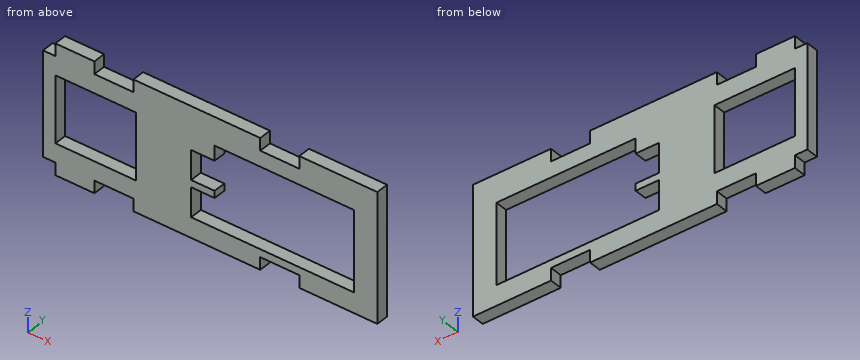
```python
from build123d import *

# Parameters (mm, degrees)
SKETCH1_W           = 20.6
SKETCH1_H           = 17
BOSS_EXTRUDE1_DEPTH = 3.17


with BuildPart() as part:
    # Sketch1 → Boss-Extrude1 (new body)
    with BuildSketch(Plane(origin=(0, 0, 0), x_dir=(1, 0, 0), z_dir=(0, 1, 0))):
        Polygon((55.67, 29.77), (55.67, 32.94), (23.17, 32.94), (23.17, 29.77), (13.17, 29.77), (13.17, 32.94), (3.17, 32.94), (3.17, 29.77), (0, 29.77), (0, 3.17), (3.17, 3.17), (3.17, 0), (13.17, 0), (13.17, 3.17), (23.17, 3.17), (23.17, 0), (55.67, 0), (55.67, 3.17), (65.67, 3.17), (65.67, 0), (85.67, 0), (85.67, 32.94), (65.67, 32.94), (65.67, 29.77), align=None)
        with Locations((13.47, 16.47)):
            Rectangle(SKETCH1_W, SKETCH1_H, mode=Mode.SUBTRACT)
        Polygon((37.97, 27.77), (43.97, 27.77), (79.67, 27.77), (79.67, 7.17), (43.97, 7.17), (43.97, 10.97), (37.97, 10.97), (37.97, 18.47), (43.97, 18.47), (43.97, 20.27), (37.97, 20.27), align=None, mode=Mode.SUBTRACT)
    extrude(amount=-BOSS_EXTRUDE1_DEPTH)


solid = part.part
```
Could you check a few things on this model? Use its own coordinates, in mm. Round coordinates to 2 decimals unless told otherwise and drop trailing zeros. Order: outer loops, then holes, each group sorted by start corner. A loop starts at its lowest first (then second) coordinate and runs counter-clockwise, first axis right, second up. Notation, with made-up numbers: (66, 54.5) -> (94, 54.5) arc R20 ccw to (94, 75.5) -> close; hole circle Ø4 at (-15.5, 48.5). An arc over 180 degrees is marked (long way). One line per question, with ' | ' between items.
Q1. I'm going to push flat-ended pins straight in: pin 1 (1.6 mm diameter, centred on x = 17.5, y = -2.5, fed in from +Z); pin 2 (1 mm diameter, centred on x = 61, y = -1.5, fed in from -Z); pin 3 (1.6 mm diameter, centred on y = -1.5, z = -31, fed in from -X); pin 4 (1.5 mm diameter, centred on y = -2.5, z = -5.5, fed in from -X). Where does each tip first touch, or does it pass through?
Computed values:
pin 1: z = -3.17 | pin 2: z = -29.77 | pin 3: x = 3.17 | pin 4: x = 0
Q2. If we section it at C-C on z = -23.5: Write out the boundary of the cut face in (x, y).
Computed values:
outline: (0, -3.17) -> (3.17, -3.17) -> (3.17, 0) -> (0, 0) -> close; (23.77, -3.17) -> (37.97, -3.17) -> (37.97, 0) -> (23.77, 0) -> close; (79.67, -3.17) -> (85.67, -3.17) -> (85.67, 0) -> (79.67, 0) -> close
Q3. If we section it at D-D on y = -0.9: Give the number of separate pieces and of enclosed holes in the cut face, plus the area to 3 significant figures.
Computed values:
separate pieces: 1 | enclosed holes: 2 | area: 1,500 mm²
Q4. If we section it at B-B on x = 41.5: Write out the boundary of the cut face in (y, z), plus the area to 3 significant figures.
Computed values:
outline: (-3.17, -32.94) -> (0, -32.94) -> (0, -27.77) -> (-3.17, -27.77) -> close; (-3.17, -20.27) -> (0, -20.27) -> (0, -18.47) -> (-3.17, -18.47) -> close; (-3.17, -10.97) -> (0, -10.97) -> (0, 0) -> (-3.17, 0) -> close | area: 56.9 mm²
Q5. If we section it at A-A on x = 18.5: Write out the boundary of the cut face in (y, z).
Computed values:
outline: (-3.17, -29.77) -> (0, -29.77) -> (0, -24.97) -> (-3.17, -24.97) -> close; (-3.17, -7.97) -> (0, -7.97) -> (0, -3.17) -> (-3.17, -3.17) -> close
Q6. If I drill on line 1 (X direction, y = -1.95, z = -24); line 2 (Z direction, x = 41, y = -0.4); line 3 (Z direction, x = 76.5, y = -2.45), over which ranges is the centre line in solid material (lowest first)? Write a range as from..to.
Computed values:
line 1: 0..3.17, 23.77..37.97, 79.67..85.67 | line 2: -32.94..-27.77, -20.27..-18.47, -10.97..0 | line 3: -32.94..-27.77, -7.17..0
